Read the model definition and answer for the solid it produces. Units are mm, in the model's axes. Face numbers are marked on the shaded views. A direction names the side the tool comes from. Coordinates: 2 decimals unless noted, no trailing zeros. Order: outer loops, then holes, each group sorted by start corner. A loop starts at its lowest first (then second) coordinate and runs counter-clockwise, first axis right, second up. Notation, with made-up numbers: M 55,86.25 L 61,86.25 A24 ccw 61,113.25 Z; hole C -36.75,55.5 d3. An arc over 180 degrees is marked long. One line per question, with ' | ' between items. Start each with the question number.
1) A tool of negligible diameter and unlimited length cuts with its end or side. For the marked faces 1, 2, 3, 4 and 5, from which of +Z, -Z, +X, -X, +Y, -Y can it reach the whole face along a straight path? Write none if from no direction.
2) Find section D-D, the plane x = 0. Write down the section's boundary in (y, z) (3 decimals).
3) Find section C-C, the plane z = -4. Write down the section's boundary in (x, y).
4) Find section B-B, the plane y = 44. Write down the section's boundary in (x, z) (3 decimals).
5) Given P1, Ø6, axis at x = -6.5, y = 44.5, coming from the +Z side; P2, Ø10, axis at y = 43, z = 9.5, coming from the -X side; P3, Ø3.5, axis at x = -11.5, z = 0, coming from the -Y side, each flat-ended and moving along its own axis, determine where each tip first touches the part or whether it passes through.
6) The mould has two halves that part along Y. Classify the marked faces 6, 7, 8 and 9: +Y half, -Y half, draft (parallel to the pull), parting line (faces both ways), or undercut.
7) Find section A-A, the plane x = -11.5. Write down the section's boundary in (y, z) (3 decimals).
8) Consider probe 1 along Z at (x, y) = (-6.4, 44) (3 decimals); probe 2 along X at (y, z) = (5.8, 0) (3 decimals); probe 3 along Z at (x, y) = (0, 5.95) (3 decimals). Determine where each line is inside the solid, lowest interval first.
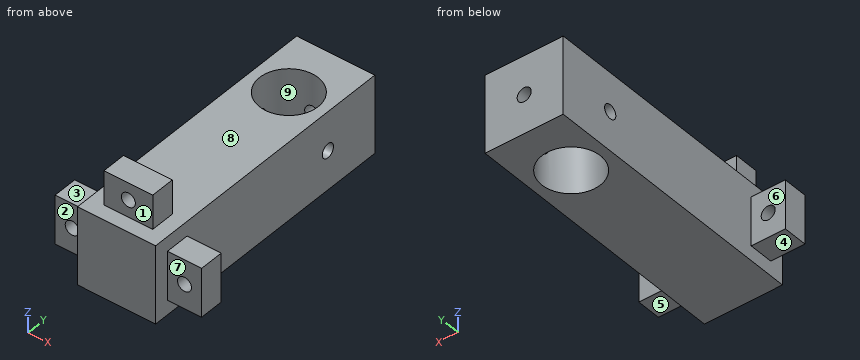
from build123d import *

# Parameters (mm, degrees)
CROQUIS1_W              = 16
CROQUIS1_H              = 16
SALIENTE_EXTRUIR1_DEPTH = 56
CORTAR_EXTRUIR1_REACH   = 18
CROQUIS2_R              = 6
CROQUIS3_R              = 1.435
CORTAR_EXTRUIR2_DEPTH   = 16
CORTAR_EXTRUIR3_REACH   = 58
CROQUIS4_R              = 1.435
CROQUIS5_W              = 10
CROQUIS5_H              = 5
SALIENTE_EXTRUIR2_DEPTH = 7
CROQUIS6_R              = 1.435
CORTAR_EXTRUIR4_DEPTH   = 5
CROQUIS7_W              = 10
CROQUIS7_H              = 5
SALIENTE_EXTRUIR3_DEPTH = 7
CORTAR_EXTRUIR5_REACH   = 10
CROQUIS8_R              = 1.435


with BuildPart() as part:
    # Croquis1 → Saliente-Extruir1 (new body)
    with BuildSketch(Plane(origin=(0, 0, 0), x_dir=(1, 0, 0), z_dir=(0, 1, 0))):
        Rectangle(CROQUIS1_W, CROQUIS1_H)
    extrude(amount=SALIENTE_EXTRUIR1_DEPTH)

    # Croquis2 → Cortar-Extruir1 (cut, up to next)
    with BuildSketch(Plane.XY.offset(8), mode=Mode.PRIVATE) as cortar_extruir1_sk1:
        with Locations((0, 44)):
            Circle(CROQUIS2_R)
    cortar_extruir1_tool1 = extrude(cortar_extruir1_sk1.sketch, amount=-CORTAR_EXTRUIR1_REACH, mode=Mode.PRIVATE) & part.part
    add(cortar_extruir1_tool1.solids().sort_by_distance((0, 44, 8))[0], mode=Mode.SUBTRACT)

    # Croquis3 → Cortar-Extruir2 (cut)
    with BuildSketch(Plane(origin=(8, 0, 0), x_dir=(0, 0, -1), z_dir=(1, 0, 0))):
        with Locations((0, 44)):
            Circle(CROQUIS3_R)
    extrude(amount=-CORTAR_EXTRUIR2_DEPTH, mode=Mode.SUBTRACT)

    # Croquis4 → Cortar-Extruir3 (cut, up to next)
    with BuildSketch(Plane(origin=(0, 56, 0), x_dir=(1, 0, 0), z_dir=(0, 1, 0)), mode=Mode.PRIVATE) as cortar_extruir3_sk1:
        Circle(CROQUIS4_R)
    cortar_extruir3_tool1 = extrude(cortar_extruir3_sk1.sketch, amount=-CORTAR_EXTRUIR3_REACH, mode=Mode.PRIVATE) & part.part
    add(cortar_extruir3_tool1.solids().sort_by_distance((0, 56, 0))[0], mode=Mode.SUBTRACT)

    # Croquis5 → Saliente-Extruir2 (add)
    with BuildSketch(Plane.ZY.offset(8)):
        with Locations((0, 5.5)):
            Rectangle(CROQUIS5_W, CROQUIS5_H)
    saliente_extruir2 = extrude(amount=SALIENTE_EXTRUIR2_DEPTH)

    # Croquis6 → Cortar-Extruir4 (cut)
    with BuildSketch(Plane(origin=(0, 8, 0), x_dir=(1, 0, 0), z_dir=(0, 1, 0))):
        with Locations((-11.5, 0)):
            Circle(CROQUIS6_R)
    cortar_extruir4 = extrude(amount=-CORTAR_EXTRUIR4_DEPTH, mode=Mode.SUBTRACT)

    # Simetría1: Saliente-Extruir2, Cortar-Extruir4 across plane
    add(saliente_extruir2.mirror(Plane(origin=(0, 0, 0), x_dir=(0, 0, 1), z_dir=(1, 0, 0))))
    add(cortar_extruir4.mirror(Plane(origin=(0, 0, 0), x_dir=(0, 0, 1), z_dir=(1, 0, 0))), mode=Mode.SUBTRACT)

    # Croquis7 → Saliente-Extruir3 (add)
    with BuildSketch(Plane.XY.offset(8)):
        with Locations((0, 5.5)):
            Rectangle(CROQUIS7_W, CROQUIS7_H)
    extrude(amount=SALIENTE_EXTRUIR3_DEPTH)

    # Croquis8 → Cortar-Extruir5 (cut, up to next)
    with BuildSketch(Plane(origin=(0, 8, 0), x_dir=(1, 0, 0), z_dir=(0, 1, 0)), mode=Mode.PRIVATE) as cortar_extruir5_sk1:
        with Locations((0, -11.5)):
            Circle(CROQUIS8_R)
    cortar_extruir5_tool1 = extrude(cortar_extruir5_sk1.sketch, amount=-CORTAR_EXTRUIR5_REACH, mode=Mode.PRIVATE) & part.part
    add(cortar_extruir5_tool1.solids().sort_by_distance((0, 8, 11.5))[0], mode=Mode.SUBTRACT)


solid = part.part
Report:
1) face 1: +Z, +X, -X, -Y | face 2: +Z, -Z, -X, -Y | face 3: +Z, -X, +Y, -Y | face 4: -Z, -X, +Y, -Y | face 5: -Z, +X, +Y, -Y
2) outline: M 0,-8 L 38,-8 L 38,8 L 8,8 L 8,10.065 L 3,10.065 L 3,8 L 0,8 Z; M 3,12.935 L 8,12.935 L 8,15 L 3,15 Z; M 50,-8 L 56,-8 L 56,-1.435 L 50,-1.435 Z; M 50,1.435 L 56,1.435 L 56,8 L 50,8 Z
3) outline: M -15,3 L -8,3 L -8,0 L 8,0 L 8,3 L 15,3 L 15,8 L 8,8 L 8,56 L -8,56 L -8,8 L -15,8 Z; hole C 0,44 d12
4) outline: M -8,-8 L -6,-8 L -6,-1.435 L -8,-1.435 Z; M -8,1.435 L -6,1.435 L -6,8 L -8,8 Z; M 6,-8 L 8,-8 L 8,-1.435 L 6,-1.435 Z; M 6,1.435 L 8,1.435 L 8,8 L 6,8 Z
5) P1: stops at z = 8 | P2: stops at x = -8 | P3: stops at y = 3
6) face 6: +Y half | face 7: -Y half | face 8: draft | face 9: undercut
7) outline: M 3,-5 L 8,-5 L 8,-1.435 L 3,-1.435 Z; M 3,1.435 L 8,1.435 L 8,5 L 3,5 Z
8) probe 1: z = -8 to -1.435, 1.435 to 8 | probe 2: x = -15 to -12.935, -10.065 to 10.065, 12.935 to 15 | probe 3: z = -8 to 10.065, 12.935 to 15
